The figure shows three views and two pictorial views of one solid part (mm, origin at its lowest corner). Answer the questions. A direction names the side the tool comes from. Coordinates: 2 decimals unless noted, no trailing zeros. Loops run counter-clockwise (first coordinate to the right, second up) from the corner with the lowest first, then second, coordinate; pieces in that order, holes last. Notation, with made-up numbers: M 80,71.5 L 117,71.5 A21 cw 117,75.5 Z; hole C 70.5,39.5 d1. An arc over 180 degrees is marked long. Answer as a JSON object with one key per item and string values. Group by question number.
1. A cutting plane is placed at A-A on x = 3. Give the vertices of the cut face in (y, z).
2. A cutting plane is placed at D-D on x = 49.5. Give the vertices of the cut face in (y, z), and give its area (3 significant figures).
3. Straight lines are drawn through the part: L1, parallel to Z at x = 50, y = 4.75; L2, parallel to X at y = 8, z = 7.25; L3, parallel to X at y = 13, z = 6.5. For each, find the intervals that lie inside material, in ascending order.
4. Given pin 1 (1 mm diameter, centred on y = 7.5, z = 7, fed in from -X); pin 2 (4.5 mm diameter, centred on x = 35.5, y = 9.5, fed in from -Z), each flat-ended and moving along its own axis, determine where each tip first touches the part or whether it passes through.
5. A cutting plane is placed at B-B on y = 12.2. Give the vertices of the cut face in (x, z), and give its area (3 significant figures).
6. A cutting plane is placed at C-C on z = 4.25. Give the vertices of the cut face in (x, y), and give its area (3 significant figures).
7. For the marked faces 1 and 2, determine the directions among +Z, -Z, +X, -X, +Y, -Y from which every point of the face is accessible in a straight line to the end or side of a thin tool.
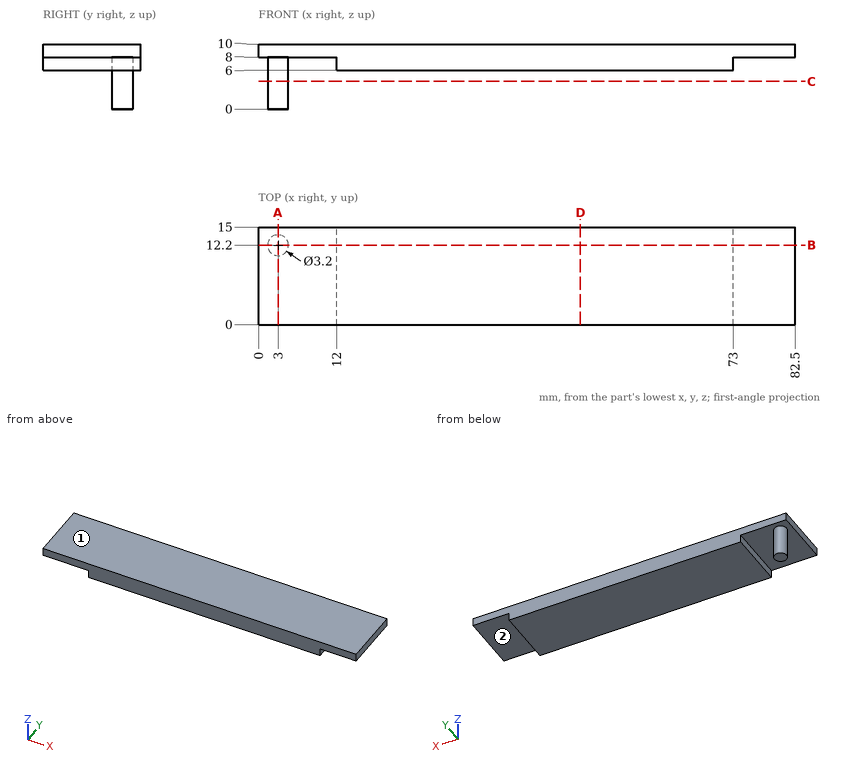
From the geometry:
{
 "1": {"outline": "M 0,8 L 10.6,8 L 10.6,0 L 13.8,0 L 13.8,8 L 15,8 L 15,10 L 0,10 Z"},
 "2": {"outline": "M 0,6 L 15,6 L 15,10 L 0,10 Z", "area": "60.0 mm²"},
 "3": {"L1": "z = 6 to 10", "L2": "x = 12 to 73", "L3": "x = 1.61 to 4.39, 12 to 73"},
 "4": {"pin 1": "stops at x = 12", "pin 2": "stops at z = 6"},
 "5": {"outline": "M 0,8 L 1.4,8 L 1.4,0 L 4.6,0 L 4.6,8 L 12,8 L 12,6 L 73,6 L 73,8 L 82.5,8 L 82.5,10 L 0,10 Z", "area": "313 mm²"},
 "6": {"outline": "C 3,12.2 d3.2", "area": "8.04 mm²"},
 "7": {"face 1": "+Z, +X, -X, +Y, -Y", "face 2": "-Z, +X, +Y, -Y"}
}
